Autodesk Inventor part; units mm, degrees
ref_plane "YZ Plane" through (0, 0, 0) normal (1, 0, 0) x (0, 1, 0)
ref_plane "XZ Plane" through (0, 0, 0) normal (0, 1, 0) x (-1, 0, 0)
ref_plane "XY Plane" through (0, 0, 0) normal (0, 0, 1) x (1, 0, 0)
sketch "スケッチ1" plane through (0, 0, 0) normal (0, 0, 1) x (1, 0, 0)
  line L0 (-122.1591, 122.1591) -> (-82.1591, 122.1591)
  line L1 (-82.1591, 122.1591) -> (-82.1591, 67.1591)
  line L2 (-82.1591, 67.1591) -> (-122.1591, 67.1591)
  line L3 (-122.1591, 67.1591) -> (-122.1591, 122.1591)
  point P0 (0, 0)
  dimension "d0" = 40
  dimension "d1" = 55
extrude "押し出し1" add sketch "スケッチ1" along normal blind 150
sketch "スケッチ4" plane through (0, 0, 150) normal (0, 0, 1) x (1, 0, 0)
  line L0 (-82.1591, 122.1591) -> (-122.1591, 122.1591)
  line L1 (-117.1591, 101.5897) -> (-92.1591, 101.5897)
  line L2 (-92.1591, 101.5897) -> (-92.1591, 122.1591)
  line L3 (-92.1591, 122.1591) -> (-117.1591, 122.1591)
  line L4 (-117.1591, 122.1591) -> (-117.1591, 101.5897)
  line L5 (-82.1591, 67.1591) -> (-82.1591, 122.1591)
  point P0 (0, 0)
  dimension "d4" = 10
  dimension "d5" = 25
extrude "押し出し2" cut sketch "スケッチ4" against normal blind 21.4
sketch "スケッチ5" plane through (0, 0, 150) normal (0, 0, 1) x (1, 0, 0)
  line L0 (-116.288, 107.2289) -> (-115.2421, 122.1591)
  line L1 (-93.2061, 122.1591) -> (-92.1591, 107.2289)
  line L2 (-95.5428, 103.9291) -> (-112.9179, 103.9291)
  line L3 (-115.2421, 122.1591) -> (-93.2061, 122.1591)
  line L4 (-112.2468, 103.9291) -> (-108.7036, 103.9291)
  line L5 (-95.5428, 103.9291) -> (-112.9179, 103.9291)
  line L6 (-92.1591, 104.7291) -> (-92.1591, 104.7291)
  line L7 (-116.2893, 104.7291) -> (-116.288, 103.9291)
  line L8 (-116.288, 103.9291) -> (-114.2025, 103.9291)
  line L9 (-92.1591, 104.7291) -> (-92.1591, 103.9291)
  line L10 (-95.5428, 103.9291) -> (-92.1591, 103.9291)
  line L11 (-114.2025, 103.9291) -> (-112.9179, 103.9291)
  line L12 (-116.2893, 104.7291) -> (-116.288, 103.9291)
  line L13 (-116.288, 103.9291) -> (-112.9179, 103.9291)
  line L14 (-92.1591, 104.7291) -> (-92.1591, 103.9291)
  line L15 (-95.5428, 103.9291) -> (-92.1591, 103.9291)
  line L16 (-92.1591, 103.9291) -> (-92.1591, 107.2289)
  line L17 (-92.1591, 103.9291) -> (-95.5428, 103.9291)
  line L18 (-95.5428, 103.9291) -> (-116.288, 103.9291)
  line L19 (-116.288, 103.9291) -> (-116.288, 104.7291)
  line L20 (-116.288, 107.2289) -> (-116.288, 104.7291)
  point P0 (0, 0)
extrude "押し出し3" cut sketch "スケッチ5" against normal blind 130
sketch "スケッチ6" plane through (0, 0, 150) normal (0, 0, 1) x (1, 0, 0)
  line L0 (-122.1591, 67.1591) -> (-82.1591, 67.1591)
  line L1 (-122.1591, 67.1591) -> (-97.1591, 67.1591)
  line L2 (-97.1591, 67.1591) -> (-97.1591, 97.1591)
  line L3 (-97.1591, 97.1591) -> (-122.1591, 97.1591)
  line L4 (-122.1591, 97.1591) -> (-122.1591, 67.1591)
  line L5 (-82.1591, 67.1591) -> (-82.1591, 122.1591)
  point P0 (0, 0)
  dimension "d10" = 30
  dimension "d11" = 15
extrude "押し出し4" cut sketch "スケッチ6" against normal blind 170
sketch "スケッチ7" plane through (-82.1591, 67.1591, 0) normal (1, 0, 0) x (0, 0, -1)
  circle A0 centre (-140.2625, 35) radius 1.65
  circle A1 centre (-107.2625, 13) radius 1.65
  circle A2 centre (-45.2625, 13) radius 1.65
  circle A3 centre (-12.2625, 35) radius 1.65
  point P0 (0, -67.1591)
  dimension "d14" = 3.3
  dimension "d15" = 3.3
  dimension "d16" = 3.3
  dimension "d17" = 3.3
extrude "押し出し5" cut sketch "スケッチ7" against normal blind 5
fillet "フィレット1" radius 2 26 edges at (-122.1591, 109.6591, 0) (-122.1591, 97.1591, 75) (-122.1591, 122.1591, 75) (-102.1591, 122.1591, 0) (-122.1591, 109.6591, 150) (-119.6591, 122.1591, 150) (-117.1591, 111.8744, 150) (-92.1591, 102.7594, 150) (-92.1591, 114.694, 150) (-87.1591, 122.1591, 150) (-92.1591, 122.1591, 139.3) (-104.6591, 101.5897, 150) (-109.6591, 97.1591, 150) (-97.1591, 82.1591, 150) (-97.1591, 67.1591, 75) (-89.6591, 67.1591, 150) (-97.1591, 82.1591, 0) (-89.6591, 67.1591, 0) (-97.1591, 97.1591, 75) (-109.6591, 97.1591, 0) (-104.2241, 122.1591, 20) (-117.1591, 122.1591, 139.3) (-116.2006, 122.1591, 128.6) (-92.6826, 122.1591, 128.6) (-115.2421, 122.1591, 74.3) (-93.2061, 122.1591, 74.3)
properties part number "structure_core_cradle"
Read the model definition and answer for the solid it produces. Units are mm, in the model's axes. A direction names the side the tool comes from. Give positions to 0.01 mm unless a question says otherwise; leave off trailing zeros. Loops run counter-clockwise (first coordinate to the right, second up) from the corner with the lowest first, then second, coordinate; pieces in that order, holes last. Notation, with made-up numbers: (28, -23) -> (79, -23) arc R10 ccw to (79, -5) -> close; hole circle Ø2 at (4, 36). An arc over 180 degrees is marked (long way). Use a Markdown table: item, result.
Q1. Determine the mould class of faces 5 (the face through (-108, 103, 128.6)), 6 (the face through (-105, 101.59, 138)), 7 (the face through (-87.159, 80, 107)) for opening direction Y: pulls with the +Y half, pulls with the -Y half, needs draft (parallel to the pull), parting line crosses it, or undercut.
Solved:
| item | result |
|---|---|
| face 5 | needs draft |
| face 6 | pulls with the +Y half |
| face 7 | undercut |
Q2. Find the intervals of material crossed by line 1 along X through (y, z) = (106, 84.5); line 2 along X through (y, z) = (113, 131); line 3 along X through (y, z) = (74, 86), in increasing order.
Solved:
| item | result |
|---|---|
| line 1 | x = -122.16 to -116.29, -92.16 to -82.16 |
| line 2 | x = -122.16 to -117.16, -92.16 to -82.16 |
| line 3 | x = -97.16 to -82.16 |
Q3. Section A-A, the plane x = -110 is taken. Determine the outline of the cut face in (y, z), then the cut area to 3 significant figures.
Solved:
| item | result |
|---|---|
| outline | (97.16, 2) arc R2 ccw to (99.16, 0) -> (120.16, 0) arc R2 ccw to (122.16, 2) -> (122.16, 18) arc R2 ccw to (120.16, 20) -> (103.93, 20) -> (103.93, 128.6) -> (101.59, 128.6) -> (101.59, 148) arc R2 ccw to (99.59, 150) -> (99.16, 150) arc R2 ccw to (97.16, 148) -> close |
| area | 1,330 mm^2 |
Q4. Each of these flat-tipped pins is pushed along its axis until it touches: pin 1 (12 mm diameter, centred on x = -99.5, z = 50.5, fed in from +Y); pin 2 (8 mm diameter, centred on x = -113, z = 94, fed in from -Y); pin 3 (8 mm diameter, centred on x = -99, y = 73.5, fed in from +Z); pin 4 (4 mm diameter, centred on y = 86, z = 21, fed in from -X). Where does it stop, or does it pass through?
Solved:
| item | result |
|---|---|
| pin 1 | stops at y = 103.93 |
| pin 2 | stops at y = 97.16 |
| pin 3 | stops at z = 150 |
| pin 4 | stops at x = -97.16 |
Q5. Section C-C, the plane z = 67.5 is taken. Determine the outline of the cut face in (x, y), then the cut area to 3 significant figures.
Solved:
| item | result |
|---|---|
| outline | (-122.16, 99.16) arc R2 ccw to (-120.16, 97.16) -> (-99.16, 97.16) arc R2 cw to (-97.16, 95.16) -> (-97.16, 69.16) arc R2 ccw to (-95.16, 67.16) -> (-82.16, 67.16) -> (-82.16, 122.16) -> (-91.06, 122.16) arc R2 ccw to (-93.06, 120.02) -> (-92.16, 107.23) -> (-92.16, 103.93) -> (-116.29, 103.93) -> (-116.29, 104.73) -> (-116.29, 107.23) -> (-115.39, 120.02) arc R2 ccw to (-117.39, 122.16) -> (-120.16, 122.16) arc R2 ccw to (-122.16, 120.16) -> close |
| area | 1,020 mm^2 |
Q6. Section B-B, the plane y = 115 is taken. Determine the outline of the cut face in (x, z), then the cut area to 3 significant figures.
Solved:
| item | result |
|---|---|
| outline | (-122.16, 2) arc R2 ccw to (-120.16, 0) -> (-82.16, 0) -> (-82.16, 150) -> (-90.16, 150) arc R2 ccw to (-92.16, 148) -> (-92.16, 128.6) -> (-92.7, 128.6) -> (-92.7, 20) -> (-115.74, 20) -> (-115.74, 128.6) -> (-117.16, 128.6) -> (-117.16, 148) arc R2 ccw to (-119.16, 150) -> (-120.16, 150) arc R2 ccw to (-122.16, 148) -> close |
| area | 2,960 mm^2 |
Q7. Section D-D, the plane y = 76 is taken. Determine the outline of the cut face in (x, z), then the cut area to 3 significant figures.
Solved:
| item | result |
|---|---|
| outline | (-97.16, 2) arc R2 ccw to (-95.16, 0) -> (-82.16, 0) -> (-82.16, 150) -> (-95.16, 150) arc R2 ccw to (-97.16, 148) -> close |
| area | 2,250 mm^2 |
Q8. A tool of negligible diameter and unlimited length cuts with its end or side. For faces 1 (the face through (-84.624, 101.527, 138.738)), 2 (the face through (-110, 97.159, 76)), 3 (the face through (-117.159, 111, 138)), 4 (the face through (-92.159, 107, 103)), from which of +Z, -Z, +X, -X, +Y, -Y can it reach the whole face along a straight path? Write none if from no direction.
Solved:
| item | result |
|---|---|
| face 1 | +X |
| face 2 | +Z, -Z, -X, -Y |
| face 3 | +Z, +Y |
| face 4 | +Z |
